Read the model definition and answer for the solid it produces. Units are mm, in the model's axes. A direction names the side the tool comes from. Coordinates: 2 decimals unless noted, no trailing zeros. Loops run counter-clockwise (first coordinate to the right, second up) from the corner with the lowest first, then second, coordinate; pieces in that order, holes last. Notation, with made-up numbers: M 82.25,64.5 L 133.25,64.5 A21 ccw 133.25,88.5 Z; hole C -30,60 d6. An arc over 180 degrees is marked long. Use one line per item in the form item = value. Start each with the question number.
1. For a pull along Y with two mould halves and no side action, classify faces 1 (the flat face through (-7.5, 287, 0)), 2 (the cylindrical face through (16.127, 283.504, -0.176)), 3 (the flat face through (-0.1, 257.5, 3.3)) as released by +Y, released by -Y, zero draft, split by the parting line, or undercut.
2. Flat-ended cylindrical pins translate along their axes: pin 1 (10 mm diameter, centred on x = 3, z = 8.5, fed in from +Y); pin 2 (5 mm diameter, centred on y = 67, z = -6, fed in from -X); pin 3 (12 mm diameter, centred on y = 23.5, z = -1, fed in from +X). Find the tip coordinate at first contact, or state that the pin passes through.
3. The part is cut by section B-B (y = 87). Give the vertices of the cut face in (x, z).
4. Find the intervals of material crossed by probe 1 along Y at (x, z) = (-0.25, 0); probe 2 along Z at (x, y) = (0, 181); probe 3 along Z at (x, y) = (-3, -53), in increasing order. Write a range as [from, to].
5. The part is cut by section A-A (y = 287.5). Give the vertices of the cut face in (x, z).
6. A tool of negligible diameter and unlimited length cuts with its end or side. For faces 4 (the flat face through (7.5, 284.5, 3)), 5 (the flat face through (25, 287, 0)), 6 (the flat face through (-0.1, -102.5, 3.3)), from which of +Z, -Z, +X, -X, +Y, -Y can it reach the whole face along a straight path? Write none if from no direction.
Autodesk Inventor part; units mm, degrees
ref_plane "YZ Plane" through (0, 0, 0) normal (1, 0, 0) x (0, 1, 0)
ref_plane "XZ Plane" through (0, 0, 0) normal (0, 1, 0) x (-1, 0, 0)
ref_plane "XY Plane" through (0, 0, 0) normal (0, 0, 1) x (1, 0, 0)
sketch "Sketch1" plane through (0, 0, 0) normal (1, 0, 0) x (0, 1, 0)
  line L0 (300, 0) -> (-300, 0)
  circle A0 centre (287.5, 0) radius 12.5
  circle A1 centre (287.5, 0) radius 4
  line L1 (287.5, 0) -> (-120, 0)
  line L2 (-120, 0) -> (-120, 3)
  line L3 (-120, 3) -> (287.5, 3)
  line L4 (287.5, 3) -> (287.5, 0)
  line L5 (257.5, 0) -> (-102.5, 0)
  line L6 (-102.5, 0) -> (-102.5, 5)
  line L7 (-102.5, 5) -> (257.5, 5)
  line L8 (257.5, 5) -> (257.5, 0)
  point P0 (0, 0)
  point P1 (-120, 0)
  point P2 (283.5, 0)
  point P3 (284.8542, 3)
  point P4 (-102.5, 0)
  point P5 (257.5, 0)
  dimension "d0" = 600
  dimension "d1" = 25
  dimension "d2" = 12.5
  dimension "d3" = 8
  dimension "d4" = 3
  dimension "d12" = 360
  dimension "d13" = 5
  dimension "d16" = 30
revolve "Revolution1" add sketch "Sketch1" angle 360 about axis through (0, 300, 0) along (0, -1, 0) picked at (277.9311, 1.2871) contours L3 A1 L0 A0 | A0 L0 L8 L3 | L8 L0 L6 L3 | L6 L0 L2 L3
extrude "Extrusion2" add sketch "Sketch1" along normal blind 25 contours A1 L0 | L0 L4 L3 A1 | L0 A1 L3 L4
extrude "Extrusion3" add sketch "Sketch1" along normal mid plane 15 contours A0 L0 A1 | L0 A1 L3 A0 | A1 L0 | L0 L4 L3 A1 | L3 A1 L0 A0 | L0 A1 L3 L4
revolve "Revolution2" add sketch "Sketch1" angle 360 about axis through (0, 287.5, 0) along (0, -1, 0) contours L8 L0 L6 L3 | L3 L6 L7 L8
sketch "Sketch2" plane through (0, 0, 0) normal (1, 0, 0) x (0, 1, 0)
  circle A0 centre (-114.1043, 0) radius 1.5
  point P0 (0, 0)
  dimension "d17" = 3
extrude "Extrusion4" cut sketch "Sketch2" along normal mid plane 15
properties part number "tierod"
Computed values:
q1.face_1 = zero draft
q1.face_2 = split by the parting line
q1.face_3 = undercut
q2.pin_1 = 299.5
q2.pin_2 = -3.57
q2.pin_3 = 5
q3.outline = C 0,0 d10
q4.probe_1 = [-120, -115.6], [-112.6, 300]
q4.probe_2 = [-5, 5]
q4.probe_3 = [-4, 4]
q5.outline = M -7.5,-12.5 L 7.5,-12.5 L 7.5,-4 L 25,-4 L 25,4 L 7.5,4 L 7.5,12.5 L -7.5,12.5 Z
q6.face_4 = +X
q6.face_5 = +Z, -Z, +X, +Y, -Y
q6.face_6 = -Y
